For this review, take the finished solid that the model builds, in its own axes (mm). A direction names the side the tool comes from. Round coordinates to 2 decimals unless told otherwise and drop trailing zeros. Order: outer loops, then holes, each group sorted by start corner. A loop starts at its lowest first (then second) coordinate and runs counter-clockwise, first axis right, second up. Notation, with made-up numbers: (12, -11) -> (31, -11) arc R23 ccw to (31, 4) -> close; hole circle Ø7 at (-1.5, -19.5). An arc over 180 degrees is marked (long way). Put each result on its own line as item: value. Start each with the question number.
```python
from build123d import *

# Parameters (mm, degrees)
SKETCH1_W            = 200
SKETCH1_H            = 90
BOSS_EXTRUDE1_DEPTH  = 3.175
CUT_EXTRUDE1_DEPTH   = 110.704515062
M3_CLEARANCE_HOLE1_D = 3.2
FILLET1_R            = 3
FILLET2_R            = 1


with BuildPart() as part:
    # Sketch1 → Boss-Extrude1 (new body)
    with BuildSketch(Plane.XY):
        Rectangle(SKETCH1_W, SKETCH1_H)
    extrude(amount=BOSS_EXTRUDE1_DEPTH)

    # Sketch2 → Cut-Extrude1 (cut, through all)
    with BuildSketch(Plane.XY.offset(3.175)):
        Polygon((-90, 33.756373771), (-90, -33.756373771), (-7.889901637, 0), align=None)
        Polygon((-82.110098363, 37), (0, 3.243626229), (82.110098363, 37), align=None)
        Polygon((90, 33.756373771), (7.889901637, 0), (90, -33.756373771), align=None)
        Polygon((-82.110098363, -37), (0, -3.243626229), (82.110098363, -37), align=None)
    extrude(amount=-CUT_EXTRUDE1_DEPTH, mode=Mode.SUBTRACT)

    # M3 Clearance Hole1 (through all)
    with Locations(Plane.XY.offset(3.175)):
        with Locations((-75, 42.61875), (75, 42.61875), (75, -42.61875), (-75, -42.61875)):
            Hole(M3_CLEARANCE_HOLE1_D / 2)

    # Fillet1
    fillet1_edges = [part.edges().sort_by_distance(p)[0] for p in [
        (-82.110098363, 37, 1.5875),
        (82.110098363, 37, 1.5875),
        (0, 3.243626229, 1.5875),
        (82.110098363, -37, 1.5875),
        (-82.110098363, -37, 1.5875),
        (0, -3.243626229, 1.5875),
        (90, 33.756373771, 1.5875),
        (90, -33.756373771, 1.5875),
        (7.889901637, 0, 1.5875),
        (-90, 33.756373771, 1.5875),
        (-7.889901637, 0, 1.5875),
        (-90, -33.756373771, 1.5875),
    ]]
    fillet(fillet1_edges, radius=FILLET1_R)

    # Fillet2
    fillet2_edges = [part.edges().sort_by_distance(p)[0] for p in [
        (100, -45, 1.5875),
        (-100, -45, 1.5875),
        (-100, 45, 1.5875),
        (100, 45, 1.5875),
    ]]
    fillet(fillet2_edges, radius=FILLET2_R)


solid = part.part
```
Item 1: Tool access review of faces 3 (the face through (50.7, 17.6, 1.6)), 4 (the face through (-24, -9, 3.175)): name each direction out of +Z, -Z, +X, -X, +Y, -Y from which nothing blocks a thin tool from reaching the whole face with its end or side.
Item 2: Consider section C-C, the plane x = 79. Write out the cut boundary in (y, z) (3 decimals), plus the area to 3 significant figures.
Item 3: Mouldability with a two-part tool opening along Y and no side actions: class faces 1 (the face through (-24, -9, 0)), 2 (the face through (-35.07, -17.66, 1.61)) as +Y half, -Y half, draft (parallel to the pull), parting line (faces both ways), or undercut.
Item 4: Consider section A-A, the plane x = -6. Write out the cut boundary in (y, z) (3 decimals), plus the area to 3 significant figures.
Item 5: Consider section B-B, the plane y = 34.5. Write out the cut boundary in (x, z) (3 decimals).
Item 6: For L1, parallel to X at y = 7.5, z = 3; L2, parallel to X at y = 22, z = 1.45; L3, parallel to Y at x = -75, z = 1.05, list the stretches that pass through material, from the lowest coordinate up.
Item 7: Consider section D-D, the plane y = 24. Write out the cut boundary in (x, z) (3 decimals).
Evaluation:
1. face 3: +Z, -Z
1. face 4: +Z, +X, -X, +Y, -Y
2. outline: (-45, 0) -> (-29.234, 0) -> (-29.234, 3.175) -> (-45, 3.175) -> close; (29.234, 0) -> (45, 0) -> (45, 3.175) -> (29.234, 3.175) -> close
2. area: 100 mm^2
3. face 1: draft
3. face 2: undercut
4. outline: (-45, 0) -> (-37, 0) -> (-37, 3.175) -> (-45, 3.175) -> close; (-5.71, 0) -> (5.71, 0) -> (5.71, 3.175) -> (-5.71, 3.175) -> close; (37, 0) -> (45, 0) -> (45, 3.175) -> (37, 3.175) -> close
4. area: 87.1 mm^2
5. outline: (-100, 0) -> (-69.881, 0) -> (-69.881, 3.175) -> (-100, 3.175) -> close; (69.881, 0) -> (100, 0) -> (100, 3.175) -> (69.881, 3.175) -> close
6. L1: x = -100 to -90, -26.13 to -10.35, 10.35 to 26.13, 90 to 100
6. L2: x = -100 to -90, -61.4 to -45.62, 45.62 to 61.4, 90 to 100
6. L3: y = -45 to -44.22, -41.02 to -27.59, 27.59 to 41.02, 44.22 to 45
7. outline: (-100, 0) -> (-90, 0) -> (-90, 3.175) -> (-100, 3.175) -> close; (-66.268, 0) -> (-50.488, 0) -> (-50.488, 3.175) -> (-66.268, 3.175) -> close; (50.488, 0) -> (66.268, 0) -> (66.268, 3.175) -> (50.488, 3.175) -> close; (90, 0) -> (100, 0) -> (100, 3.175) -> (90, 3.175) -> close
